Study the drawing (mm; zero at the part's minimum x, y, z) and answer. A direction names the side the tool comes from. Round coordinates to 2 decimals unless told otherwise and drop trailing zeros. Write each loop counter-clockwise with the first axis right and the second up, starting at its lowest first coordinate (ties: lowest second). Pieces come first, ordered by that corner, then holes. Notation, with made-up numbers: (-33.75, 86.5) - (-14.75, 86.5) arc R25 ccw to (-14.75, 105.5) - close; hole circle Ø6 at (87.25, -35). An arc over 180 degrees is marked (long way). Use one line per item in the form item = value. Start each with the question number.
1) The part is cut by section B-B, the plane z = 28. Give the vertices of the cut face in (x, y).
2) For the marked faces 4, 5 and 6, determine the directions among +Z, -Z, +X, -X, +Y, -Y from which every point of the face is accessible in a straight line to the end or side of a thin tool.
3) Consider line 1 along Z through (x, y) = (13, 23.5); line 2 along Y through (x, z) = (26, 48); line 3 along Y through (x, z) = (2.3, 11). Determine where each line is inside the solid, lowest interval first. Write a range as from..to.
4) The part is cut by section C-C, the plane y = 8.5. Count the separate pieces of the cut face and the enclosed holes in it, plus the area to 3 significant figures.
5) Each of these flat-tipped pins is pushed along its axis until it touches: pin 1 (5.5 mm diameter, centred on x = 3, z = 29, fed in from +Y); pin 2 (4 mm diameter, centred on x = 14, z = 43.5, fed in from -Y); pin 3 (5 mm diameter, centred on y = 21, z = 54.5, fed in from -X). Where does it stop, or does it pass through?
6) For a pull along Y with two mould halves and no side action, classify the marked faces 1, 2 and 3 as released by +Y, released by -Y, zero draft, split by the parting line, or undercut.
7) The part is cut by section D-D, the plane y = 18.25. Give the vertices of the cut face in (x, z), plus the area to 3 significant figures.
8) The part is cut by section A-A, the plane y = 3. Give the vertices of the cut face in (x, z), plus the area to 3 significant figures.
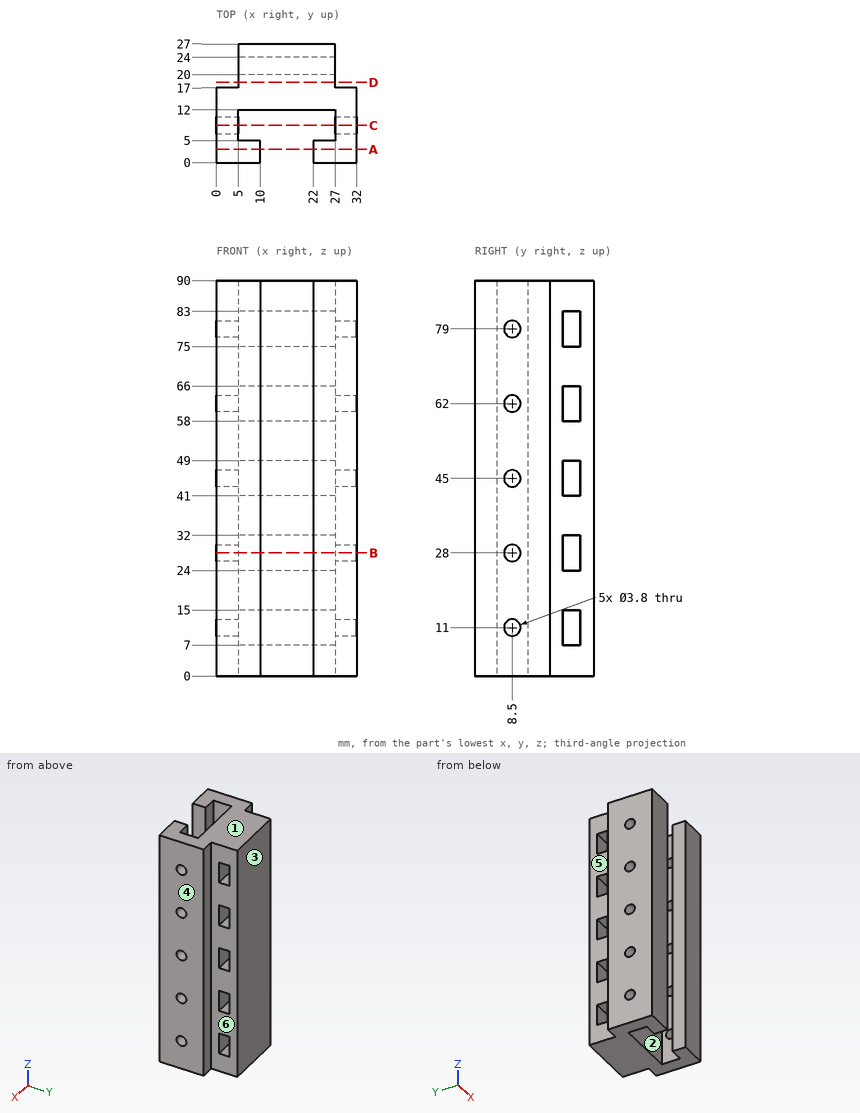
Geometry results:
q1.outline = (0, 0) - (10, 0) - (10, 5) - (5, 5) - (5, 6.6) - (0, 6.6) - close; (0, 10.4) - (5, 10.4) - (5, 12) - (27, 12) - (27, 10.4) - (32, 10.4) - (32, 17) - (27, 17) - (27, 20) - (5, 20) - (5, 17) - (0, 17) - close; (5, 24) - (27, 24) - (27, 27) - (5, 27) - close; (22, 0) - (32, 0) - (32, 6.6) - (27, 6.6) - (27, 5) - (22, 5) - close
q2.face_4 = +Z, -Z, +X, +Y, -Y
q2.face_5 = +Z, -Z, -X, +Y
q2.face_6 = +Z, -Z, +X, +Y
q3.line_1 = 0..7, 15..24, 32..41, 49..58, 66..75, 83..90
q3.line_2 = 0..5, 12..20, 24..27
q3.line_3 = 0..6.6, 10.4..17
q4.separate_pieces = 12
q4.enclosed_holes = 0
q4.area = 710 mm2
q5.pin_1 = 27
q5.pin_2 = 12
q5.pin_3 = 5
q6.face_1 = zero draft
q6.face_2 = undercut
q6.face_3 = released by +Y
q7.outline = (5, 0) - (27, 0) - (27, 90) - (5, 90) - close
q7.area = 1,980 mm2
q8.outline = (0, 0) - (10, 0) - (10, 90) - (0, 90) - close; (22, 0) - (32, 0) - (32, 90) - (22, 90) - close
q8.area = 1,800 mm2
